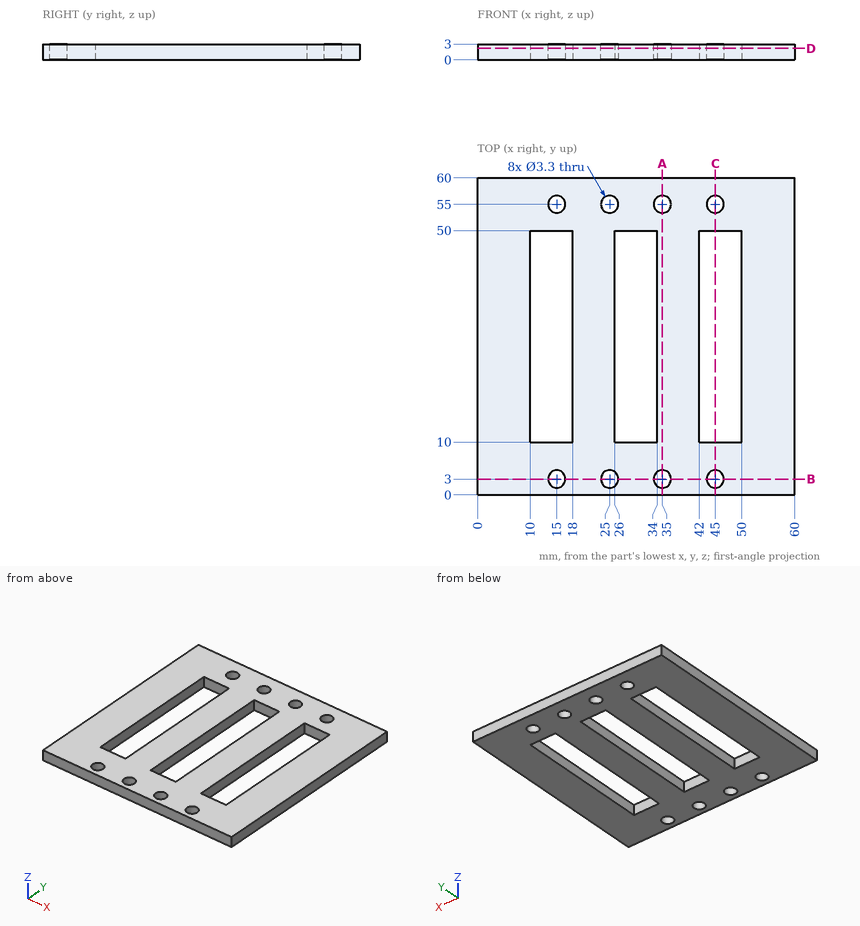
Check sheet for the drawn part. Datum: minimum x, y, z corner. Units: mm. Give positions to 0.01 mm unless a question says otherwise; leave off trailing zeros. Order: outer loops, then holes, each group sorted by start corner. A loop starts at its lowest first (then second) coordinate and runs counter-clockwise, first axis right, second up. Notation, with made-up numbers: (71.25, 39) - (86.25, 39) arc R26 ccw to (86.25, 70) - close; hole circle Ø1 at (55, 30). An arc over 180 degrees is marked (long way). Write item = value, one per line. Start each with the question number.
1) Section check D-D (z = 2.15). Count the separate pieces of the cut face and the enclosed holes in it, then the cut area to 3 significant figures.
2) Section check B-B (y = 3). Enter the section's corners in (x, z), then the cut area to 3 significant figures.
3) Scan lines: L1, parallel to X at y = 29, z = 2.65; L2, parallel to Y at x = 29, z = 0.8; L3, parallel to Y at x = 35, z = 2.1. Record each from-to range of solid material in increasing order.
4) Section check A-A (x = 35). Enter the section's corners in (y, z).
5) Section check C-C (x = 45). Enter the section's corners in (y, z).
Geometry check:
q1.separate_pieces = 1
q1.enclosed_holes = 11
q1.area = 2,570 mm2
q2.outline = (0, 0) - (13.35, 0) - (13.35, 3) - (0, 3) - close; (16.65, 0) - (23.35, 0) - (23.35, 3) - (16.65, 3) - close; (26.65, 0) - (33.35, 0) - (33.35, 3) - (26.65, 3) - close; (36.65, 0) - (43.35, 0) - (43.35, 3) - (36.65, 3) - close; (46.65, 0) - (60, 0) - (60, 3) - (46.65, 3) - close
q2.area = 140 mm2
q3.L1 = 0 to 10, 18 to 26, 34 to 42, 50 to 60
q3.L2 = 0 to 10, 50 to 60
q3.L3 = 0 to 1.35, 4.65 to 53.35, 56.65 to 60
q4.outline = (0, 0) - (1.35, 0) - (1.35, 3) - (0, 3) - close; (4.65, 0) - (53.35, 0) - (53.35, 3) - (4.65, 3) - close; (56.65, 0) - (60, 0) - (60, 3) - (56.65, 3) - close
q5.outline = (0, 0) - (1.35, 0) - (1.35, 3) - (0, 3) - close; (4.65, 0) - (10, 0) - (10, 3) - (4.65, 3) - close; (50, 0) - (53.35, 0) - (53.35, 3) - (50, 3) - close; (56.65, 0) - (60, 0) - (60, 3) - (56.65, 3) - close
